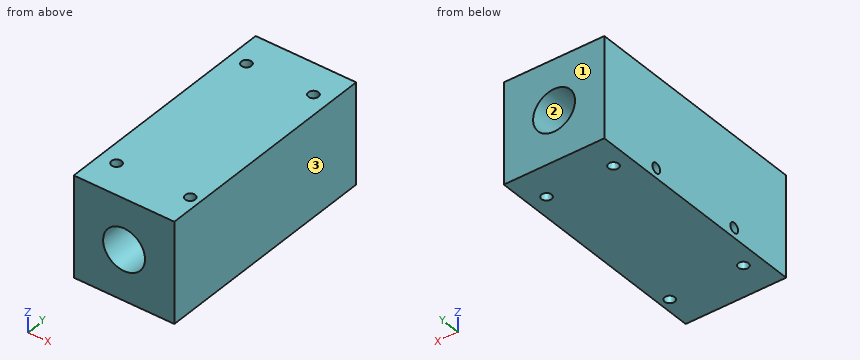
from build123d import *

# Parameters (mm, degrees)
ESBO_O1_W                = 30
ESBO_O1_H                = 70
RESSALTO_EXTRUS_O1_DEPTH = 30
ESBO_O3_R                = 6.255
CORTE_EXTRUS_O2_DEPTH    = 82.853527719
ESBO_O4_R                = 1.5
CORTE_EXTRUS_O3_DEPTH    = 82.853527719
ESBO_O5_R                = 1.5
CORTE_EXTRUS_O4_DEPTH    = 10


with BuildPart() as part:
    # Esboço1 → Ressalto-extrusão1 (new body)
    with BuildSketch(Plane.XY):
        with Locations((-15, 35)):
            Rectangle(ESBO_O1_W, ESBO_O1_H)
    extrude(amount=RESSALTO_EXTRUS_O1_DEPTH)

    # Esboço3 → Corte-extrusão2 (cut, through all)
    with BuildSketch(Plane(origin=(0, 70, 0), x_dir=(1, 0, 0), z_dir=(0, 1, 0))):
        with Locations(Location((-15, -15, 0), (0, 0, 270))):
            Circle(ESBO_O3_R)
    extrude(amount=-CORTE_EXTRUS_O2_DEPTH, mode=Mode.SUBTRACT)

    # Esboço4 → Corte-extrusão3 (cut, through all)
    with BuildSketch(Plane(origin=(0, 0, 0), x_dir=(-1, 0, 0), z_dir=(0, 0, -1))):
        with Locations((5, 60)):
            Circle(ESBO_O4_R)
        with Locations((3, 10)):
            Circle(ESBO_O4_R)
        with Locations((25, 60)):
            Circle(ESBO_O4_R)
        with Locations((25, 10)):
            Circle(ESBO_O4_R)
    extrude(amount=-CORTE_EXTRUS_O3_DEPTH, mode=Mode.SUBTRACT)

    # Esboço5 → Corte-extrusão4 (cut)
    with BuildSketch(Plane.ZY.offset(30)):
        with Locations((2.924479503, 50)):
            Circle(ESBO_O5_R)
        with Locations((2.924479503, 20)):
            Circle(ESBO_O5_R)
    extrude(amount=-CORTE_EXTRUS_O4_DEPTH, mode=Mode.SUBTRACT)


solid = part.part
Geometry check sheet. Reference: the model listing, model coordinates, mm. Face numbers are marked on the shaded views. Round coordinates to 2 decimals unless told otherwise and drop trailing zeros. Loops run counter-clockwise (first coordinate to the right, second up) from the corner with the lowest first, then second, coordinate; pieces in that order, holes last. Notation, with made-up numbers: (81.5, -11) -> (92.5, -11) arc R12 cw to (92.5, -6) -> close; hole circle Ø10 at (67.25, -27.75). An arc over 180 degrees is marked (long way). Answer as a JSON object with one key per item and string values. Group by question number.
Item 1: Thickness scan on line 1 along Y through (x, z) = (-25, 17.75); line 2 along X through (y, z) = (46.5, 15) (3 decimals); line 3 along X through (y, z) = (59, 1.5). Record the ranges inside material, lowest first.
Item 2: Cross-section at D-D, the plane y = 20. Record the cut outline in (x, z) (3 decimals), plus the area to 3 significant figures.
Item 3: Cross-section at C-C, the plane x = -25. Record the cut outline in (y, z), plus the area to 3 significant figures.
Item 4: Cross-section at A-A, the plane y = 60. Record the cut outline in (x, z) (3 decimals).
Item 5: Cross-section at B-B, the plane z = 15. Record the cut outline in (x, y) (3 decimals).
Item 6: Release check for a two-part mould opening along X. For the marked faces 1, 2 and 3 record: pulls with the +X half, pulls with the -X half, needs draft (parallel to the pull), parting line crosses it, or undercut.
Item 7: Depth check by flat-ended pin: pin 1 Ø10 at (x, y) = (-10.5, 9) entering from -Z; pin 2 Ø0.9 at (y, z) = (49.5, 2.5) entering from -X. Enter the tip coordinate at first touch or a pass-through.
Determined:
{
 "1": {"line 1": "y = 0 to 8.5, 11.5 to 58.5, 61.5 to 70", "line 2": "x = -30 to -21.255, -8.745 to 0", "line 3": "x = -30 to -26.12, -23.88 to -6.12, -3.88 to 0"},
 "2": {"outline": "(-30, 0) -> (0, 0) -> (0, 30) -> (-30, 30) -> (-30, 4.424) -> (-20, 4.424) -> (-20, 1.424) -> (-30, 1.424) -> close; hole circle Ø12.51 at (-15, 15)", "area": "747 mm²"},
 "3": {"outline": "(0, 0) -> (8.5, 0) -> (8.5, 30) -> (0, 30) -> close; (11.5, 0) -> (58.5, 0) -> (58.5, 30) -> (11.5, 30) -> close; (61.5, 0) -> (70, 0) -> (70, 30) -> (61.5, 30) -> close; hole circle Ø3 at (20, 2.92); hole circle Ø3 at (50, 2.92)", "area": "1,910 mm²"},
 "4": {"outline": "(-30, 0) -> (-26.5, 0) -> (-26.5, 30) -> (-30, 30) -> close; (-23.5, 0) -> (-6.5, 0) -> (-6.5, 30) -> (-23.5, 30) -> close; (-3.5, 0) -> (0, 0) -> (0, 30) -> (-3.5, 30) -> close; hole circle Ø12.51 at (-15, 15)"},
 "5": {"outline": "(-30, 0) -> (-21.255, 0) -> (-21.255, 70) -> (-30, 70) -> close; (-8.745, 0) -> (0, 0) -> (0, 70) -> (-8.745, 70) -> close; hole circle Ø3 at (-25, 10); hole circle Ø3 at (-25, 60); hole circle Ø3 at (-5, 60); hole circle Ø3 at (-3, 10)"},
 "6": {"face 1": "needs draft", "face 2": "undercut", "face 3": "pulls with the +X half"},
 "7": {"pin 1": "stops at z = 0", "pin 2": "stops at x = -20"}
}
